The model under review builds one solid part; all positions refer to its coordinate system, in mm. Face numbers are marked on the shaded views. A direction names the side the tool comes from. Give positions to 0.01 mm unless a question says otherwise; leave off trailing zeros. Order: outer loops, then holes, each group sorted by start corner. A loop starts at its lowest first (then second) coordinate and runs counter-clockwise, first axis right, second up.
```python
from build123d import *

# Parameters (mm, degrees)
F0_R     = 9.525
F0_R_2   = 4.960938
F1_DEPTH = 1.7145
F0_R_3   = 3.81
F2_DEPTH = 5.08
F3_R     = 1.905


with BuildPart() as f1:
    # F0 (on Top) → F1 (new body)
    with BuildSketch(Plane.XY):
        Circle(F0_R)
        Circle(F0_R_2, mode=Mode.SUBTRACT)
    extrude(amount=F1_DEPTH)

    # F0 (on Top) → F2 (join)
    with BuildSketch(Plane.XY):
        Circle(F0_R_2)
        Circle(F0_R_3, mode=Mode.SUBTRACT)
    extrude(amount=F2_DEPTH)

    # F3
    f3_edges = [f1.edges().sort_by_distance(p)[0] for p in [
        (-3.81, 0, 0),
    ]]
    fillet(f3_edges, radius=F3_R)


solid = f1.part
```
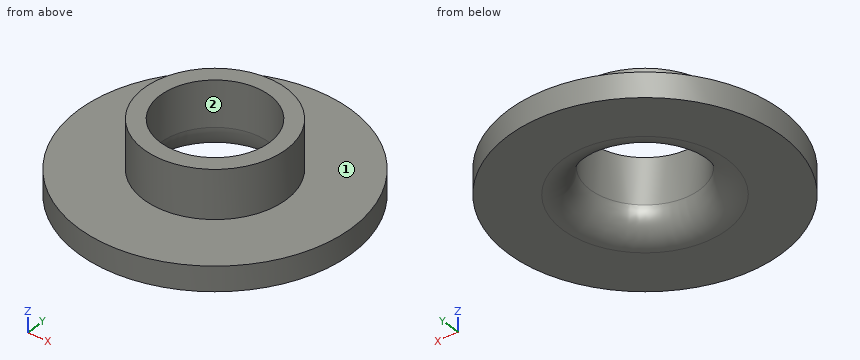
Item 1: For the marked faces 1 and 2, list the 3-axis set-ups (+Z, -Z, +X, -X, +Y, -Y) from which the entire face can be reached by the end or side of a thin tool; tool diameter is ignored.
Values found:
face 1: +Z
face 2: +Z, -Z
Item 2: Take a section at C-C (z = 2.7). Give the boundary of the cut face in (x, y), and give its area (3 significant figures).
Values found:
outline: circle Ø9.92 at (0, 0); hole circle Ø7.62 at (0, 0)
area: 31.7 mm2
Item 3: Take a section at A-A (y = 0). Give the boundary of the cut face in (x, z) (1 decimal).
Values found:
outline: (-9.5, 0) - (-5.7, 0) arc R1.9 ccw to (-3.8, 1.9) - (-3.8, 5.1) - (-5, 5.1) - (-5, 1.7) - (-9.5, 1.7) - close; (3.8, 1.9) arc R1.9 ccw to (5.7, 0) - (9.5, 0) - (9.5, 1.7) - (5, 1.7) - (5, 5.1) - (3.8, 5.1) - close
Item 4: For line 1 (Y direction, x = 0, z = 3.15); line 2 (Y direction, x = 3.25, z = 0.85); line 3 (X direction, y = -0.75, z = 4.4), list the stretches that pass through material, from the lowest coordinate up.
Values found:
line 1: y = -4.96 to -3.81, 3.81 to 4.96
line 2: y = -8.95 to -2.55, 2.55 to 8.95
line 3: x = -4.9 to -3.74, 3.74 to 4.9
Item 5: Take a section at D-D (y = 8.75). Give the boundary of the cut face in (x, z), and give its area (3 significant figures).
Values found:
outline: (-3.76, 0) - (3.76, 0) - (3.76, 1.71) - (-3.76, 1.71) - close
area: 12.9 mm2
Item 6: Clearance check with flat-ended pins moving along their axes: pin 1 Ø2 at (x, z) = (-0.5, 3) entering from -Y; pin 2 Ø4.5 at (x, y) = (0, 0) entering from +Z; pin 3 Ø1.5 at (x, y) = (-4.5, 5) entering from -Z; pin 4 Ø1.5 at (x, z) = (3, 2) entering from +Y. State where each tip first meets the part, or that it passes through.
Values found:
pin 1: stops at y = -4.96
pin 2: passes through
pin 3: stops at z = 0
pin 4: stops at y = 9.24
